from build123d import *

# Parameters (mm, degrees)
EXTRUDE_1_DEPTH          = 34
EXTRUDE_1_DEPTH_BACK     = 3
EXTRUDE_START            = -3
EXTRUDE_2_DEPTH          = 37
PATTERN_CIRCULAR_1_COUNT = 6


# Read off the part's stored shape, not the designer's step: 切除-旋转-薄壁1
with BuildPart() as part:
    # 草图2 → 凸台-拉伸1 (new, two sides: drawn at the far end of the back side and taken through both)
    with BuildSketch(Plane(origin=(0, 0, 0), x_dir=(1, 0, 0), z_dir=(0, 1, 0)).offset(-EXTRUDE_1_DEPTH_BACK)):
        with BuildLine():
            ThreePointArc((-2.491861702, -9.684556018), (-1.255874162, -9.920825575), (0, -10))
            Line((0, -10), (0, 10))
            ThreePointArc((0, 10), (-9.920825575, 1.255874162), (-2.491861702, -9.684556018))
        make_face()
        with BuildLine():
            Line((0, 10), (0, -10))
            ThreePointArc((0, -10), (1.255874162, -9.920825575), (2.491861702, -9.684556018))
            ThreePointArc((2.491861702, -9.684556018), (7.903120175, -6.127045903), (10, 0))
            ThreePointArc((10, 0), (7.071067812, 7.071067812), (0, 10))
        make_face()
    extrude(amount=EXTRUDE_1_DEPTH + EXTRUDE_1_DEPTH_BACK)

    # 草图2<3> → 凸台-拉伸2 (add)
    with BuildSketch(Plane(origin=(0, 0, 0), x_dir=(1, 0, 0), z_dir=(0, 1, 0)).offset(EXTRUDE_START)):
        with BuildLine():
            ThreePointArc((-1.5, -12.409673646), (-0.751358578, -12.477397977), (0, -12.5))
            Line((0, -12.5), (0, -10))
            ThreePointArc((0, -10), (-1.255874162, -9.920825575), (-2.491861702, -9.684556018))
            Line((-2.491861702, -9.684556018), (-1.5, -12.409673646))
        make_face()
        with BuildLine():
            Line((0, -10), (0, -12.5))
            ThreePointArc((0, -12.5), (0.751358578, -12.477397977), (1.5, -12.409673646))
            Line((1.5, -12.409673646), (2.491861702, -9.684556018))
            ThreePointArc((2.491861702, -9.684556018), (1.255874162, -9.920825575), (0, -10))
        make_face()
    extrude_2 = extrude(amount=EXTRUDE_2_DEPTH)

    # 阵列(圆周)1: 凸台-拉伸2 ×6 about axis
    pattern_circular_1_axis = Axis((0, 0, 0), (0, 1, 0))
    for i in range(1, PATTERN_CIRCULAR_1_COUNT):
        add(extrude_2.rotate(pattern_circular_1_axis, i * 360 / PATTERN_CIRCULAR_1_COUNT))

    # 草图3 → 切除-旋转1 (revolve, cut)
    with BuildSketch(Plane(origin=(0, 0, 0), x_dir=(0, 0, -1), z_dir=(1, 0, 0)), mode=Mode.PRIVATE) as cut_revolve_1_sk:
        Polygon((-12.5, 0), (-8.5, 0), (-8.5, 8), (-12.5, 9.07179677), align=None)
    revolve(cut_revolve_1_sk.sketch.rotate(Axis((0, -3, 0), (0, 1, 0)), 353.107897421), axis=Axis((0, -3, 0), (0, 1, 0)), mode=Mode.SUBTRACT)

    # 切除-旋转-薄壁1 outline → 切除-旋转-薄壁1 (revolve, cut)
    with BuildSketch(Plane.XY):
        with BuildLine():
            ThreePointArc((0, 34), (7.828815855, 31.378325603), (12.500000004, 24.570714202))
            Line((12.500000004, 24.570714202), (12.500000004, 34))
            Line((12.500000004, 34), (0, 34))
        make_face()
    revolve(axis=Axis((0, 0, 0), (0, 1, 0)), mode=Mode.SUBTRACT)


solid = part.part
Could you check a few things on this model? Use its own coordinates, in mm. A direction names the side the tool comes from. Give positions to 0.01 mm unless a question says otherwise; leave off trailing zeros. Order: outer loops, then holes, each group sorted by start corner. A loop starts at its lowest first (then second) coordinate and runs counter-clockwise, first axis right, second up.
1. Suppose I cut it at B-B (y = 25). Write out the boundary of the cut face in (x, z), plus the area to 3 significant figures.
Answers below:
outline: (-11.4, -4.79) arc R12.37 ccw to (-9.85, -7.48) - (-7.14, -7) arc R10 ccw to (-2.49, -9.68) - (-1.55, -12.27) arc R12.37 ccw to (1.55, -12.27) - (2.49, -9.68) arc R10 ccw to (7.14, -7) - (9.85, -7.48) arc R12.37 ccw to (11.4, -4.79) - (9.63, -2.68) arc R10 ccw to (9.63, 2.68) - (11.4, 4.79) arc R12.37 ccw to (9.85, 7.48) - (7.14, 7) arc R10 ccw to (2.49, 9.68) - (1.55, 12.27) arc R12.37 ccw to (-1.55, 12.27) - (-2.49, 9.68) arc R10 ccw to (-7.14, 7) - (-9.85, 7.48) arc R12.37 ccw to (-11.4, 4.79) - (-9.63, 2.68) arc R10 ccw to (-9.63, -2.68) - close
area: 372 mm2
2. Suppose I cut it at D-D (y = 7). Write out the boundary of the cut face in (x, z).
Answers below:
outline: circle Ø17 at (0, 0)
3. I need wall thicknesses on L1, parallel to Z at x = 0.25, y = 15.5; L2, parallel to Z at x = 7, y = 9.5; L3, parallel to Y at x = 0.25, z = -9.75. Which ranges of each line are inside material? Lowest first, please.
Answers below:
L1: z = -12.5 to 12.5
L2: z = -7.14 to 7.14
L3: y = -3 to 0, 8.34 to 29.6
4. Suppose I cut it at C-C (y = 31.5). Write out the boundary of the cut face in (x, z), plus the area to 3 significant figures.
Answers below:
outline: circle Ø15.33 at (0, 0)
area: 185 mm2
5. Thinking about a two-plate mould opening in Z: for faces 5 (the flat face through (-10.55, -1.52, 3.78)), 6 (the flat face through (-10.55, 18.71, 3.78)), 7 (the flat face through (2.003, -1.521, -11.028)), 8 (the cylindrical face through (1.562, 4.056, 8.355)), which applies, +Z half, -Z half, draft (parallel to the pull), parting line (faces both ways), or undercut?
Answers below:
face 5: undercut
face 6: undercut
face 7: -Z half
face 8: parting line
6. For pin 1 (8 mm diameter, centred on y = 19, z = -0.5, fed in from +X); pin 2 (7 mm diameter, centred on x = -4, z = -6, fed in from +Y); pin 3 (3 mm diameter, centred on y = 27.5, z = -1, fed in from -X), each with a flat end and sliding along its axis, tell me the tip position at first contact or that it passes through.
Answers below:
pin 1: stops at x = 11.16
pin 2: stops at y = 33.46
pin 3: stops at x = -10
7. Suppose I cut it at A-A (y = 15). Write out the boundary of the cut face in (x, z), plus the area to 3 significant figures.
Answers below:
outline: (-11.5, -4.91) arc R12.5 ccw to (-10, -7.5) - (-7.14, -7) arc R10 ccw to (-2.49, -9.68) - (-1.5, -12.41) arc R12.5 ccw to (1.5, -12.41) - (2.49, -9.68) arc R10 ccw to (7.14, -7) - (10, -7.5) arc R12.5 ccw to (11.5, -4.91) - (9.63, -2.68) arc R10 ccw to (9.63, 2.68) - (11.5, 4.91) arc R12.5 ccw to (10, 7.5) - (7.14, 7) arc R10 ccw to (2.49, 9.68) - (1.5, 12.41) arc R12.5 ccw to (-1.5, 12.41) - (-2.49, 9.68) arc R10 ccw to (-7.14, 7) - (-10, 7.5) arc R12.5 ccw to (-11.5, 4.91) - (-9.63, 2.68) arc R10 ccw to (-9.63, -2.68) - close
area: 374 mm2
8. Which directions (+Z, -Z, +X, -X, +Y, -Y) give clear straight access to the entire face, cutting with the end or side of a thin tool? Please do faces 1 (the flat face through (-8.55, -1.52, -7.25)), 2 (the conical face through (1.608, 8.067, 8.601)), 3 (the flat face through (10.55, -1.52, -3.78)), 4 (the flat face through (8.55, -1.52, 7.25)).
Answers below:
face 1: -Z, +Y, -Y
face 2: none
face 3: +X, +Y, -Y
face 4: +Z, +Y, -Y
